from build123d import *

# Parameters (mm, degrees)
EXTRUDE_1_DEPTH = 60
FILLET_1_R      = 2
SKETCH_2_W      = 60
SKETCH_2_H      = 5.5
EXTRUDE_2_DEPTH = 30
FILLET_3_R      = 2
SKETCH_3_W      = 2
SKETCH_3_H      = 46
EXTRUDE_3_DEPTH = 48
SKETCH_4_W      = 2
SKETCH_4_H      = 18
EXTRUDE_4_DEPTH = 13
SKETCH_5_W      = 2
SKETCH_5_H      = 18
EXTRUDE_5_DEPTH = 13
FILLET_4_R      = 1
FILLET_5_R      = 2.5


with BuildPart() as part:
    # 草圖1 → 填料-伸長1 (new body)
    with BuildSketch(Plane(origin=(0, 0, 0), x_dir=(0, 0, -1), z_dir=(1, 0, 0))):
        Polygon((-42.254416961, 29.533568905), (-42.254416961, -20.466431095), (7.745583039, -20.466431095), (7.745583039, 11.533568905), (18.745583039, 11.533568905), (18.745583039, 21.533568905), (5.745583039, 11.533568905), (5.745583039, -18.466431095), (-40.254416961, -18.466431095), (-40.254416961, 29.533568905), align=None)
    extrude(amount=EXTRUDE_1_DEPTH)

    # 圓角1
    fillet_1_edges = [part.edges().sort_by_distance(p)[0] for p in [
        (30, 11.533568905, -7.745583039),
    ]]
    fillet(fillet_1_edges, radius=FILLET_1_R)

    # 草圖2 → 填料-伸長2 (add)
    with BuildSketch(Plane.XZ.offset(-11.533568905)):
        with Locations((30, -12.495583039)):
            Rectangle(SKETCH_2_W, SKETCH_2_H)
    extrude(amount=EXTRUDE_2_DEPTH)

    # 圓角3
    fillet_3_edges = [part.edges().sort_by_distance(p)[0] for p in [
        (30, 11.533568905, -15.245583039),
    ]]
    fillet(fillet_3_edges, radius=FILLET_3_R)

    # 草圖3 → 填料-伸長3 (add)
    with BuildSketch(Plane(origin=(0, -18.466431095, 0), x_dir=(1, 0, 0), z_dir=(0, 1, 0))):
        with Locations((1, -17.254416961)):
            Rectangle(SKETCH_3_W, SKETCH_3_H)
        with Locations((59, -17.254416961)):
            Rectangle(SKETCH_3_W, SKETCH_3_H)
    extrude(amount=EXTRUDE_3_DEPTH)

    # 草圖4 → 填料-伸長4 (add)
    with BuildSketch(Plane(origin=(0, 0, -5.745583039), x_dir=(-1, 0, 0), z_dir=(0, 0, -1))):
        with Locations((-1, 20.533568905)):
            Rectangle(SKETCH_4_W, SKETCH_4_H)
    extrude(amount=EXTRUDE_4_DEPTH)

    # 草圖5 → 填料-伸長5 (add)
    with BuildSketch(Plane(origin=(0, 0, -5.745583039), x_dir=(-1, 0, 0), z_dir=(0, 0, -1))):
        with Locations((-59, 20.533568905)):
            Rectangle(SKETCH_5_W, SKETCH_5_H)
    extrude(amount=EXTRUDE_5_DEPTH)

    # 圓角4
    fillet_4_edges = [part.edges().sort_by_distance(p)[0] for p in [
        (30, 11.533568905, -18.745583039),
    ]]
    fillet(fillet_4_edges, radius=FILLET_4_R)

    # 圓角5
    fillet_5_edges = [part.edges().sort_by_distance(p)[0] for p in [
        (60, -18.466431095, -12.495583039),
        (30, -18.466431095, -9.745583039),
        (30, -18.466431095, -15.245583039),
        (0, -18.466431095, -12.495583039),
    ]]
    fillet(fillet_5_edges, radius=FILLET_5_R)


solid = part.part
Input: part model. Units: mm. Frame: model coordinates. A direction names the side the tool comes from. Give positions to 0.01 mm unless a question says otherwise; leave off trailing zeros. Loops run counter-clockwise (first coordinate to the right, second up) from the corner with the lowest first, then second, coordinate; pieces in that order, holes last. Notation, with made-up numbers: (63.25, 22.25) - (122.25, 22.25) arc R17 cw to (122.25, 55.25) - close; hole circle Ø4 at (8, 63). An arc over 180 degrees is marked (long way). Use CSV: the item, a comma, the result in double quotes. Start each with the question number.
Item 1: Section D-D on y = 20.5. Return loops of the section in (x, z).
Item 2: Section B-B on x = 27. Return loops of the section in (y, z), then the cut area to 3 significant figures.
Item 3: Mould query, pull axis Z, two halves, no side actions, for faces 5 (the flat face through (30, -20.466, 18)), 6 (the cylindrical face through (30.42, 10.932, -15.816)), 7 (the flat face through (58, 5, 18)). Classes: pulls with the +Z half, pulls with the -Z half, needs draft (parallel to the pull), parting line crosses it, or undercut.
Item 4: Section C-C on z = 25.5. Return loops of the section in (x, y).
Item 5: Reachability of faces 1 (the flat face through (30, -3, -5.746)), 2 (the flat face through (30, -3, -15.246)), 3 (the flat face through (30, -2, -9.746)), 4 (the cylindrical face through (0.44, -17.38, -12.46)) from +Z, -Z, +X, -X, +Y, -Y: full face, straight path, thin tool, end or side. Return the list, or none.
Item 6: Line query: line 1 (Z direction, x = 56, y = 5); line 2 (X direction, y = -15, z = 9); line 3 (Z direction, x = 23, y = -17). Output: solid intervals per line, ascending.
Item 7: Contact query for flat-ended pins moving along their axis: P1, Ø7.5, axis at x = 29.5, y = -8, coming from the -Z side; P2, Ø10, axis at x = 15, z = -12, coming from the +Y side; P3, Ø12, axis at x = 38, z = 32.5, coming from the +Y side. Output: stop coordinate, or through.
Item 8: Section A-A on y = -12. Return loops of the section in (x, z).
Ans:
1,outline,"(0, -18.75) - (60, -18.75) - (60, 42.25) - (0, 42.25) - close; hole (2, -17.4) - (58, -17.4) - (58, 40.25) - (2, 40.25) - close"
2,outline,"(-20.47, -7.75) - (9.53, -7.75) arc R2 cw to (11.53, -9.75) - (-15.97, -9.75) arc R2.5 ccw to (-18.47, -12.25) - (-18.47, -12.75) arc R2.5 ccw to (-15.97, -15.25) - (9.53, -15.25) arc R2 cw to (11.53, -17.25) - (11.53, -17.75) arc R1 ccw to (12.53, -18.75) - (21.53, -18.75) - (11.53, -5.75) - (-18.47, -5.75) - (-18.47, 40.25) - (29.53, 40.25) - (29.53, 42.25) - (-20.47, 42.25) - close"
2,area,"485 mm2"
3,face 5,"needs draft"
3,face 6,"pulls with the -Z half"
3,face 7,"undercut"
4,outline,"(0, -20.47) - (60, -20.47) - (60, 29.53) - (58, 29.53) - (58, -18.47) - (2, -18.47) - (2, 29.53) - (0, 29.53) - close"
5,face 1,"+Y"
5,face 2,"-Z, +X, -X, -Y"
5,face 3,"+X, -X, -Y"
5,face 4,"-Z, -X, -Y"
6,line 1,"z = -15.25 to -9.75, -7.75 to -5.75, 40.25 to 42.25"
6,line 2,"x = 0 to 2, 58 to 60"
6,line 3,"z = -15.02 to -9.97, -7.75 to -5.75, 40.25 to 42.25"
7,P1,"stops at z = -15.25"
7,P2,"stops at y = 20.19"
7,P3,"stops at y = -18.47"
8,outline,"(0, -15.25) - (60, -15.25) - (60, -9.75) - (0, -9.75) - close; (0, -7.75) - (60, -7.75) - (60, 42.25) - (0, 42.25) - close; hole (2, -5.75) - (58, -5.75) - (58, 40.25) - (2, 40.25) - close"
